Geometry: final body of the model. Coordinates: model frame, mm. Face numbers are marked on the shaded views. A direction names the side the tool comes from. Give positions to 0.01 mm unless a question says otherwise; leave off trailing zeros. Order: outer loops, then holes, each group sorted by start corner. A loop starts at its lowest first (then second) coordinate and runs counter-clockwise, first axis right, second up. Notation, with made-up numbers: (-36.75, 15) -> (-8.75, 15) arc R26 ccw to (-8.75, 34) -> close; hole circle Ø10 at (70, 41.5). An arc over 180 degrees is marked (long way). One line per question, with ' | ' between items.
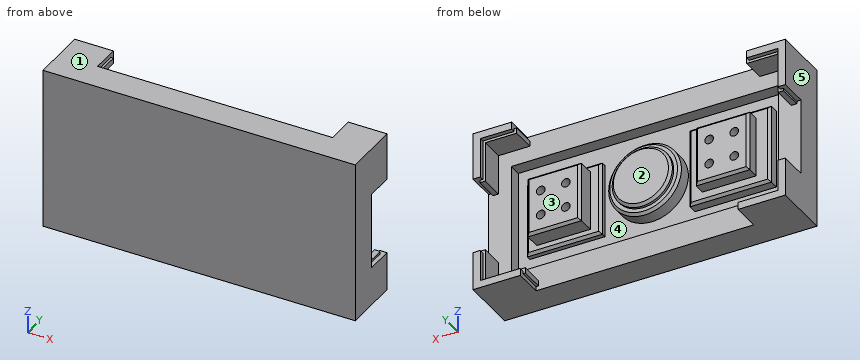
Autodesk Inventor part; units mm, degrees
ref_plane "YZ Plane" through (0, 0, 0) normal (1, 0, 0) x (0, 1, 0)
ref_plane "XZ Plane" through (0, 0, 0) normal (0, 1, 0) x (-1, 0, 0)
ref_plane "XY Plane" through (0, 0, 0) normal (0, 0, 1) x (1, 0, 0)
sketch "Sketch1" plane through (0, 0, 0) normal (0, 1, 0) x (-1, 0, 0)
  line L0 (62.25, -32.4) -> (-62.25, -32.4)
  line L1 (-62.25, -32.4) -> (-62.25, 32.4)
  line L2 (-62.25, 32.4) -> (62.25, 32.4)
  line L3 (62.25, 32.4) -> (62.25, -32.4)
  point P0 (0, 0)
  point P1 (62.25, 0)
  point P2 (0, -32.4)
  dimension "d0" = 64.8
  dimension "d2" = 124.5
extrude "Extrusion1" add sketch "Sketch1" along normal blind 11.45
sketch "Sketch2" plane through (0, 11.45, 0) normal (0, 1, 0) x (1, 0, 0)
  line L0 (62.25, 32.4) -> (-62.25, 32.4)
  line L1 (-62.25, 32.4) -> (-62.25, -32.4)
  line L2 (-62.25, -32.4) -> (62.25, -32.4)
  line L3 (62.25, -32.4) -> (62.25, 32.4)
  line L4 (-62.25, -13.55) -> (-62.25, -32.4)
  line L5 (-62.25, -32.4) -> (-46.85, -32.4)
  line L6 (-46.85, -32.4) -> (-46.85, -29.5)
  line L7 (-46.85, -29.5) -> (-59.35, -29.5)
  line L8 (-59.35, -29.5) -> (-59.35, -13.55)
  line L9 (-59.35, -13.55) -> (-62.25, -13.55)
  line L10 (62.25, -13.55) -> (59.35, -13.55)
  line L11 (59.35, -13.55) -> (59.35, -29.5)
  line L12 (59.35, -29.5) -> (46.85, -29.5)
  line L13 (46.85, -29.5) -> (46.85, -32.4)
  line L14 (62.25, -32.4) -> (62.25, -13.55)
  line L15 (46.85, -32.4) -> (62.25, -32.4)
  line L16 (43.4, 32.4) -> (43.4, 29.5)
  line L17 (43.4, 29.5) -> (59.35, 29.5)
  line L18 (62.25, 32.4) -> (43.4, 32.4)
  line L19 (59.35, 29.5) -> (59.35, 17)
  line L20 (59.35, 17) -> (62.25, 17)
  line L21 (62.25, 17) -> (62.25, 32.4)
  line L22 (-62.25, 17) -> (-59.35, 17)
  line L23 (-59.35, 17) -> (-59.35, 29.5)
  line L24 (-59.35, 29.5) -> (-43.4, 29.5)
  line L25 (-43.4, 29.5) -> (-43.4, 32.4)
  line L26 (-62.25, 32.4) -> (-62.25, 17)
  line L27 (-43.4, 32.4) -> (-62.25, 32.4)
  point P0 (0, 0)
  dimension "d5" = 18.85
  dimension "d7" = 15.4
  dimension "d8" = 2.9
  dimension "d9" = 2.9
  dimension "d10" = 18.85
  dimension "d11" = 2.9
  dimension "d12" = 2.9
  dimension "d13" = 15.4
  dimension "d21" = 15.4
  dimension "d22" = 18.85
  dimension "d23" = 2.9
  dimension "d24" = 2.9
  dimension "d28" = 15.4
  dimension "d29" = 2.9
  dimension "d30" = 2.9
  dimension "d31" = 18.85
extrude "Extrusion2" add sketch "Sketch2" along normal blind 11.3 contours L3 L20 L19 L17 L16 L0 | L25 L24 L23 L22 L1 L0 | L3 L2 L13 L12 L11 L10 | L9 L8 L7 L6 L2 L1
sketch "Sketch3" plane through (0, 11.45, 0) normal (0, 1, 0) x (1, 0, 0)
  line L0 (43.4, 32.4) -> (-43.4, 32.4)
  line L1 (-62.25, 17) -> (-62.25, -13.55)
  line L2 (-46.85, -32.4) -> (46.85, -32.4)
  line L3 (62.25, -13.55) -> (62.25, 17)
  line L4 (-53.25, 22.4) -> (53.25, 22.4)
  line L5 (53.25, 22.4) -> (53.25, -22.4)
  line L6 (53.25, -22.4) -> (-53.25, -22.4)
  line L7 (-53.25, -22.4) -> (-53.25, 22.4)
  point P0 (0, 0)
  dimension "d41" = 9
  dimension "d42" = 9
  dimension "d43" = 10
  dimension "d44" = 10
extrude "Extrusion3" cut sketch "Sketch3" against normal blind 5.1
sketch "Sketch4" plane through (0, 6.35, 0) normal (0, 1, 0) x (1, 0, 0)
  line L0 (-53.25, -22.4) -> (-53.25, 22.4)
  line L1 (-49.65, 15.75) -> (-17.15, 15.75)
  line L2 (-17.15, 15.75) -> (-17.15, -15.75)
  line L3 (-17.15, -15.75) -> (-49.65, -15.75)
  line L4 (-49.65, -15.75) -> (-49.65, 15.75)
  line L5 (43.4, 32.4) -> (-43.4, 32.4)
  point P0 (0, 0)
  dimension "d47" = 32.5
  dimension "d49" = 31.5
  dimension "d50" = 16.65
  dimension "d51" = 3.6
extrude "Extrusion4" add sketch "Sketch4" along normal blind 4.6
sketch "Sketch5" plane through (0, 10.95, 0) normal (0, 1, 0) x (1, 0, 0)
  line L0 (-17.15, 15.75) -> (-49.65, 15.75)
  line L1 (-49.65, 15.75) -> (-49.65, -15.75)
  line L2 (-44.1, 11.95) -> (-22.7, 11.95)
  line L3 (-22.7, 11.95) -> (-22.7, -11.95)
  line L4 (-22.7, -11.95) -> (-44.1, -11.95)
  line L5 (-44.1, -11.95) -> (-44.1, 11.95)
  point P0 (0, 0)
  point P1 (-33.4, 11.95)
  point P2 (-33.4, 15.75)
  point P3 (-44.1, 0)
  point P4 (-49.65, 0)
  dimension "d54" = 21.4
  dimension "d56" = 23.9
extrude "Extrusion5" add sketch "Sketch5" along normal blind 5.5
sketch "Sketch6" plane through (0, 6.35, 0) normal (0, 1, 0) x (1, 0, 0)
  line L0 (53.25, 22.4) -> (53.25, -22.4)
  line L1 (18.73, 14.8) -> (48.73, 14.8)
  line L2 (48.73, 14.8) -> (48.73, -14.8)
  line L3 (48.73, -14.8) -> (18.73, -14.8)
  line L4 (18.73, -14.8) -> (18.73, 14.8)
  point P0 (0, 0)
  point P1 (18.73, 0)
  dimension "d59" = 29.6
  dimension "d61" = 30
  dimension "d62" = 4.52
extrude "Extrusion6" add sketch "Sketch6" along normal blind 2.8
sketch "Sketch7" plane through (0, 9.15, 0) normal (0, 1, 0) x (1, 0, 0)
  line L0 (48.73, 14.8) -> (18.73, 14.8)
  line L1 (18.73, 14.8) -> (18.73, -14.8)
  line L2 (23.03, 11.95) -> (44.43, 11.95)
  line L3 (44.43, 11.95) -> (44.43, -11.95)
  line L4 (44.43, -11.95) -> (23.03, -11.95)
  line L5 (23.03, -11.95) -> (23.03, 11.95)
  point P0 (0, 0)
  point P1 (23.03, 0)
  point P2 (18.73, 0)
  point P3 (33.73, 11.95)
  point P4 (33.73, 14.8)
  dimension "d65" = 21.4
  dimension "d67" = 23.9
extrude "Extrusion7" add sketch "Sketch7" along normal blind 7.3
sketch "Sketch8" plane through (0, 11.45, 0) normal (0, 1, 0) x (1, 0, 0)
  line L0 (62.25, -13.55) -> (62.25, 17)
  line L1 (-60.55, -12.55) -> (-60.55, -13.55)
  line L2 (-60.55, -13.55) -> (-59.35, -13.55)
  line L3 (-59.35, -13.55) -> (-59.35, -29.5)
  line L4 (-59.35, -29.5) -> (-46.85, -29.5)
  line L5 (-46.85, -29.5) -> (-46.85, -30.7)
  line L6 (-46.85, -30.7) -> (-45.85, -30.7)
  line L7 (-45.85, -30.7) -> (-45.85, -28.5)
  line L8 (-45.85, -28.5) -> (-58.35, -28.5)
  line L9 (-58.35, -28.5) -> (-58.35, -12.55)
  line L10 (-58.35, -12.55) -> (-60.55, -12.55)
  line L11 (-59.35, -13.55) -> (-62.25, -13.55)
  line L12 (-59.35, -29.5) -> (-59.35, -13.55)
  line L13 (-46.85, -29.5) -> (-59.35, -29.5)
  line L14 (-46.85, -32.4) -> (-46.85, -29.5)
  line L15 (60.55, 16) -> (60.55, 17)
  line L16 (60.55, 17) -> (59.35, 17)
  line L17 (59.35, 17) -> (59.35, 29.5)
  line L18 (59.35, 29.5) -> (43.4, 29.5)
  line L19 (43.4, 29.5) -> (43.4, 30.7)
  line L20 (43.4, 30.7) -> (42.4, 30.7)
  line L21 (42.4, 30.7) -> (42.4, 28.5)
  line L22 (42.4, 28.5) -> (58.35, 28.5)
  line L23 (58.35, 28.5) -> (58.35, 16)
  line L24 (58.35, 16) -> (60.55, 16)
  line L25 (43.4, 29.5) -> (59.35, 29.5)
  line L26 (59.35, 29.5) -> (59.35, 17)
  line L27 (59.35, 17) -> (62.25, 17)
  line L28 (43.4, 32.4) -> (43.4, 29.5)
  line L29 (-60.55, 16) -> (-58.35, 16)
  line L30 (-58.35, 16) -> (-58.35, 28.5)
  line L31 (-58.35, 28.5) -> (-42.4, 28.5)
  line L32 (-42.4, 28.5) -> (-42.4, 30.7)
  line L33 (-42.4, 30.7) -> (-43.4, 30.7)
  line L34 (-43.4, 30.7) -> (-43.4, 29.5)
  line L35 (-43.4, 29.5) -> (-59.35, 29.5)
  line L36 (-59.35, 29.5) -> (-59.35, 17)
  line L37 (-59.35, 17) -> (-60.55, 17)
  line L38 (-60.55, 17) -> (-60.55, 16)
  line L39 (-59.35, 29.5) -> (-43.4, 29.5)
  line L40 (-59.35, 17) -> (-59.35, 29.5)
  line L41 (-43.4, 29.5) -> (-43.4, 32.4)
  line L42 (-62.25, 17) -> (-59.35, 17)
  line L43 (60.55, -12.55) -> (58.35, -12.55)
  line L44 (58.35, -12.55) -> (58.35, -28.5)
  line L45 (58.35, -28.5) -> (45.85, -28.5)
  line L46 (45.85, -28.5) -> (45.85, -30.7)
  line L47 (45.85, -30.7) -> (46.85, -30.7)
  line L48 (46.85, -30.7) -> (46.85, -29.5)
  line L49 (46.85, -29.5) -> (59.35, -29.5)
  line L50 (59.35, -29.5) -> (59.35, -13.55)
  line L51 (59.35, -13.55) -> (60.55, -13.55)
  line L52 (60.55, -13.55) -> (60.55, -12.55)
  line L53 (59.35, -13.55) -> (59.35, -29.5)
  line L54 (62.25, -13.55) -> (59.35, -13.55)
  line L55 (59.35, -29.5) -> (46.85, -29.5)
  line L56 (46.85, -29.5) -> (46.85, -32.4)
  point P0 (0, 0)
  dimension "d70" = 1
  dimension "d72" = 1
  dimension "d73" = 1
  dimension "d74" = 1
  dimension "d76" = 2.2
  dimension "d77" = 2.2
  dimension "d78" = 1
  dimension "d79" = 1
  dimension "d80" = 1
  dimension "d81" = 1
  dimension "d82" = 2.2
  dimension "d83" = 2.2
  dimension "d86" = 2.2
  dimension "d87" = 1
  dimension "d88" = 1
  dimension "d89" = 1
  dimension "d90" = 1
  dimension "d91" = 2.2
  dimension "d92" = 2.2
  dimension "d93" = 1
  dimension "d94" = 1
  dimension "d95" = 1
  dimension "d96" = 1
  dimension "d97" = 2.2
extrude "Extrusion8" add sketch "Sketch8" along normal blind 9.5
sketch "Sketch10" plane through (0, 6.35, 0) normal (0, 1, 0) x (1, 0, 0)
  circle A0 centre (0, 0) radius 14.5
  dimension "d133" = 29
extrude "Extrusion10" add sketch "Sketch10" along normal blind 6
sketch "Sketch11" plane through (0, 12.35, 0) normal (0, 1, 0) x (1, 0, 0)
  circle A0 centre (0, 0) radius 12
  dimension "d137" = 24
extrude "Extrusion11" add sketch "Sketch11" along normal blind 2
chamfer "Chamfer1" distance 1 angle 45 4 edges at (44.43, 16.45, 0) (33.73, 16.45, 11.95) (23.03, 16.45, 0) (33.73, 16.45, -11.95)
chamfer "Chamfer2" distance 1 angle 45 4 edges at (-33.4, 16.45, -11.95) (-44.1, 16.45, 0) (-33.4, 16.45, 11.95) (-22.7, 16.45, 0)
chamfer "Chamfer3" distance 1 angle 45 4 edges at (-33.4, 10.95, 15.75) (-49.65, 10.95, 0) (-33.4, 10.95, -15.75) (-17.15, 10.95, 0)
chamfer "Chamfer4" distance 1 angle 45 4 edges at (33.73, 9.15, -14.8) (18.73, 9.15, 0) (33.73, 9.15, 14.8) (48.73, 9.15, 0)
sketch "Sketch12" plane through (0, 16.45, 0) normal (0, 1, 0) x (1, 0, 0)
  line L0 (23.03, 11.95) -> (23.03, -11.95)
  point P0 (0, 0)
  point P1 (38.73, -5)
  point P2 (28.73, -5)
  point P3 (28.73, 5)
  point P4 (38.73, 5)
  point P5 (-38.1211, 5.7215)
  point P6 (-28.8217, 5.7215)
  point P7 (-28.8217, -4.174)
  point P8 (-38.1211, -5)
  dimension "d153" = 10
  dimension "d155" = 10
  dimension "d157" = 5
  dimension "d159" = 5.7
hole "Hole1" at (38.73, 16.45, 5) at (28.73, 16.45, 5) at (28.73, 16.45, -5) at (38.73, 16.45, -5) direction (0, -1, 0) diameter 3.459 depth 7 tip angle 118
sketch "Sketch14" plane through (0, 16.45, 0) normal (0, 1, 0) x (1, 0, 0)
  line L0 (-44.1, 11.95) -> (-44.1, -11.95)
  point P0 (0, 0)
  point P1 (-38.4, 5)
  point P2 (-28.4, 5)
  point P3 (-28.4, -5)
  point P4 (-38.4, -5)
  dimension "d167" = 10
  dimension "d169" = 10
  dimension "d170" = 5
  dimension "d171" = 5.7
hole "Hole2" at (-38.4, 16.45, -5) at (-28.4, 16.45, -5) at (-28.4, 16.45, 5) at (-38.4, 16.45, 5) direction (0, -1, 0) diameter 3.459 depth 7 tip angle 118
chamfer "Chamfer5" distance 1 angle 45 2 edges at (-12, 14.35, 0) (-14.5, 12.35, 0)
equation "\"d0\" = BtDp"
equation "\"d2\" = BtWd"
equation "\"d3\" = ModHt"
equation "\"d5\" = TopOutSh"
equation "\"d7\" = TopOutLn"
equation "\"d8\" = TopOutDp"
equation "\"d9\" = d8"
equation "\"d10\" = d5"
equation "\"d11\" = d9"
equation "\"d12\" = d9"
equation "\"d13\" = d7"
equation "\"d21\" = d25"
equation "\"d22\" = d26"
equation "\"d23\" = d27"
equation "\"d24\" = d23"
equation "\"d28\" = d32"
equation "\"d29\" = d33"
equation "\"d30\" = d33"
equation "\"d31\" = d34"
equation "\"d39\" = TopHoldHt"
equation "\"d41\" = LedgeSh"
equation "\"d42\" = d41"
equation "\"d43\" = LedgeLn"
equation "\"d44\" = d43"
equation "\"d45\" = InPdDp"
equation "\"d47\" = RedLeadPedesWd"
equation "\"d49\" = RedLeadPedesDp"
equation "\"d50\" = 0.5 * BtDp - 0.5 * RedLeadPedesDp"
equation "\"d51\" = RedLeadPedesGap"
equation "\"d52\" = RedLeadPedesHt"
equation "\"d54\" = RedLeadWd"
equation "\"d56\" = RedLeadDp"
equation "\"d57\" = RedLeadHt"
equation "\"d59\" = CyanLeadPedesWd"
equation "\"d61\" = CyanLeadPedesDp"
equation "\"d62\" = CyanLeadPedesGap"
equation "\"d63\" = CyanLeadPedesHt"
equation "\"d65\" = CyanLeadWd"
equation "\"d67\" = CyanLeadDp"
equation "\"d68\" = CyanLeadHt"
equation "\"d70\" = InCapHldWd"
equation "\"d72\" = d70"
equation "\"d73\" = d70"
equation "\"d74\" = d73"
equation "\"d76\" = InCapHldDp"
equation "\"d77\" = d76"
equation "\"d78\" = d84"
equation "\"d79\" = d78"
equation "\"d80\" = d78"
equation "\"d81\" = d80"
equation "\"d82\" = d85"
equation "\"d83\" = d82"
equation "\"d32\" = d35"
equation "\"d33\" = d36"
equation "\"d34\" = d37"
equation "\"d36\" = d38"
properties part number "batteryCellTop" material "Aluminum 6061"
1) Contact query for flat-ended pins moving along their axis: pin 1 Ø6 at (x, z) = (6.5, 24.5) entering from -Y; pin 2 Ø0.8 at (y, z) = (17, -16.5) entering from -X; pin 3 Ø8 at (y, z) = (20, -7) entering from -X; pin 4 Ø3 at (x, z) = (-25.5, 5.5) entering from +Y. Output: stop coordinate, or through.
Check result:
pin 1: stops at y = 0 | pin 2: stops at x = -60.55 | pin 3: stops at x = -43.55 | pin 4: stops at y = 16.45
2) Section A-A on x = 0. Return loops of the section in (y, z).
Check result:
outline: (0, -32.4) -> (11.45, -32.4) -> (11.45, -22.4) -> (6.35, -22.4) -> (6.35, -14.5) -> (11.35, -14.5) -> (12.35, -13.5) -> (12.35, -12) -> (13.35, -12) -> (14.35, -11) -> (14.35, 11) -> (13.35, 12) -> (12.35, 12) -> (12.35, 13.5) -> (11.35, 14.5) -> (6.35, 14.5) -> (6.35, 22.4) -> (11.45, 22.4) -> (11.45, 32.4) -> (0, 32.4) -> close
3) Section B-B on x = -21.5. Return loops of the section in (y, z).
Check result:
outline: (0, -32.4) -> (11.45, -32.4) -> (11.45, -22.4) -> (6.35, -22.4) -> (6.35, -15.75) -> (9.95, -15.75) -> (10.95, -14.75) -> (10.95, 14.75) -> (9.95, 15.75) -> (6.35, 15.75) -> (6.35, 22.4) -> (11.45, 22.4) -> (11.45, 32.4) -> (0, 32.4) -> close
4) Material intervals for probe 1 along Z at (x, y) = (38.73, 14.25); probe 2 along X at (y, z) = (14.5, -5); probe 3 along X at (y, z) = (9, -9), sorted ascending. Write a range as from..to.
Check result:
probe 1: z = -11.95..-6.73, -3.27..3.27, 6.73..11.95 | probe 2: x = -44.1..-40.13, -36.67..-30.13, -26.67..-22.7, 23.03..27, 30.46..37, 40.46..44.43 | probe 3: x = -62.25..-53.25, -49.65..-17.15, -11.37..11.37, 19.58..47.88, 53.25..62.25
5) Pull-direction query (X, two-part tool) for the marked faces 3, 4 and 5; classes: +X half, -X half, draft (parallel to the pull), parting line (faces both ways), or undercut.
Check result:
face 3: draft | face 4: undercut | face 5: -X half
6) Set-up query: the marked faces 1 and 2. Return all of +Z, -Z, +X, -X, +Y, -Y with unobstructed straight access to the full face (end or side cutting, diameter ignored); none if empty.
Check result:
face 1: +Z, +X, -X, +Y, -Y | face 2: +Z, -Z, +Y
